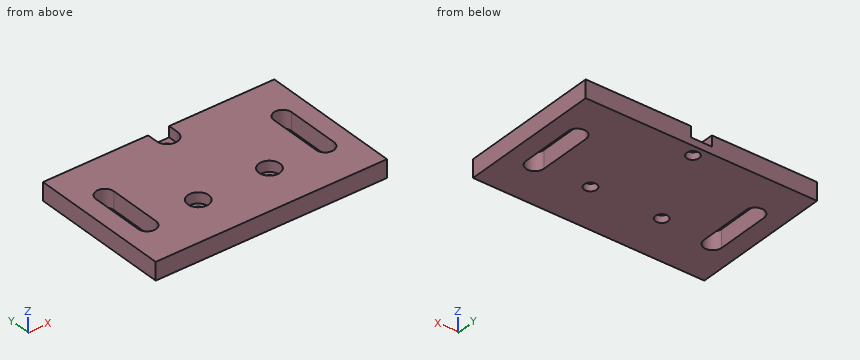
from build123d import *

# Parameters (mm, degrees)
F0_W     = 65
F0_H     = 40
F0_R     = 1.75
F1_DEPTH = 5
F2_R     = 2.95
F2_R_2   = 1.75
F3_DEPTH = 3


with BuildPart() as f1:
    # F0 (on Top) → F1 (new body)
    with BuildSketch(Plane.XY):
        Rectangle(F0_W, F0_H)
        with Locations((-10, -6.7)):
            Circle(F0_R, mode=Mode.SUBTRACT)
        with Locations((10, -6.7)):
            Circle(F0_R, mode=Mode.SUBTRACT)
        with BuildLine():
            ThreePointArc((-22.5, -7.5), (-25, -10), (-27.5, -7.5))
            Line((-27.5, -7.5), (-27.5, 7.5))
            ThreePointArc((-27.5, 7.5), (-25, 10), (-22.5, 7.5))
            Line((-22.5, 7.5), (-22.5, -7.5))
        make_face(mode=Mode.SUBTRACT)
        with BuildLine():
            ThreePointArc((27.5, -7.5), (25, -10), (22.5, -7.5))
            Line((22.5, -7.5), (22.5, 7.5))
            ThreePointArc((22.5, 7.5), (25, 10), (27.5, 7.5))
            Line((27.5, 7.5), (27.5, -7.5))
        make_face(mode=Mode.SUBTRACT)
        with Locations((0, 17)):
            Circle(F0_R, mode=Mode.SUBTRACT)
    extrude(amount=F1_DEPTH)

    # F2 (on face) → F3 (cut)
    with BuildSketch(Plane.XY.offset(5)):
        with Locations((10, -6.7)):
            Circle(F2_R)
        with Locations((10, -6.7)):
            Circle(F2_R_2, mode=Mode.SUBTRACT)
        with Locations((-10, -6.7)):
            Circle(F2_R_2)
        with Locations((-10, -6.7)):
            Circle(F2_R)
        with Locations((-10, -6.7)):
            Circle(F2_R_2, mode=Mode.SUBTRACT)
        with BuildLine():
            Line((-2.949923, 20), (-2.949923, 17.021281))
            ThreePointArc((-2.949923, 17.021281), (0, 14.05), (2.949923, 17.021281))
            Line((2.949923, 17.021281), (2.949923, 20))
            Line((2.949923, 20), (-2.949923, 20))
        make_face()
        with Locations((0, 17)):
            Circle(F2_R_2, mode=Mode.SUBTRACT)
    extrude(amount=-F3_DEPTH, mode=Mode.SUBTRACT)


solid = f1.part
Can you work these out from the model? Positions are in its coordinate system, mm. Coordinates: 2 decimals unless noted, no trailing zeros. Loops run counter-clockwise (first coordinate to the right, second up) from the corner with the lowest first, then second, coordinate; pieces in that order, holes last. Notation, with made-up numbers: (63, -23.75) - (97, -23.75) arc R19 cw to (97, -7.75) - close; hole circle Ø6 at (52.25, 54.5). An arc over 180 degrees is marked (long way). Answer as a JSON object with one key per item and string values. Group by question number.
Item 1: If we section it at D-D (z = 4.3): List the corners of the cut face in (x, y) for me, plus the area to 3 significant figures.
Item 2: For pin 1 (1.8 mm diameter, centred on x = -1, y = 15.5, fed in from +Z), with a flat end and sliding along its axis, tell me the tip position at first contact or that it passes through.
Item 3: If I drill on L1, parallel to X at y = 6.5, z = 2.5; L2, parallel to Y at x = -10, z = 3.4; L3, parallel to Y at x = 10, z = 0.9, over which ranges is the centre line in solid material (lowest first)? Write a range as from..to.
Item 4: If we section it at B-B (x = 0): List the corners of the cut face in (y, z) for me, plus the area to 3 significant figures.
Item 5: If we section it at C-C (y = 6): List the corners of the cut face in (x, z) for me, plus the area to 3 significant figures.
Item 6: If we section it at A-A (y = -6.7): List the corners of the cut face in (x, z) for me.
Returned:
{
 "1": {"outline": "(-32.5, -20) - (32.5, -20) - (32.5, 20) - (2.95, 20) - (2.95, 17.02) arc R2.95 cw (long way) to (-2.95, 17.02) - (-2.95, 20) - (-32.5, 20) - close; hole (-27.5, -7.5) arc R2.5 ccw to (-22.5, -7.5) - (-22.5, 7.5) arc R2.5 ccw to (-27.5, 7.5) - close; hole circle Ø5.9 at (-10, -6.7); hole circle Ø5.9 at (10, -6.7); hole (22.5, -7.5) arc R2.5 ccw to (27.5, -7.5) - (27.5, 7.5) arc R2.5 ccw to (22.5, 7.5) - close", "area": "2,320 mm²"},
 "2": {"pin 1": "stops at z = 2"},
 "3": {"L1": "x = -32.5..-27.5, -22.5..22.5, 27.5..32.5", "L2": "y = -20..-9.65, -3.75..20", "L3": "y = -20..-8.45, -4.95..20"},
 "4": {"outline": "(-20, 0) - (15.25, 0) - (15.25, 2) - (14.05, 2) - (14.05, 5) - (-20, 5) - close; (18.75, 0) - (20, 0) - (20, 2) - (18.75, 2) - close", "area": "175 mm²"},
 "5": {"outline": "(-32.5, 0) - (-27.5, 0) - (-27.5, 5) - (-32.5, 5) - close; (-22.5, 0) - (22.5, 0) - (22.5, 5) - (-22.5, 5) - close; (27.5, 0) - (32.5, 0) - (32.5, 5) - (27.5, 5) - close", "area": "275 mm²"},
 "6": {"outline": "(-32.5, 0) - (-27.5, 0) - (-27.5, 5) - (-32.5, 5) - close; (-22.5, 0) - (-11.75, 0) - (-11.75, 2) - (-12.95, 2) - (-12.95, 5) - (-22.5, 5) - close; (-8.25, 0) - (8.25, 0) - (8.25, 2) - (7.05, 2) - (7.05, 5) - (-7.05, 5) - (-7.05, 2) - (-8.25, 2) - close; (11.75, 0) - (22.5, 0) - (22.5, 5) - (12.95, 5) - (12.95, 2) - (11.75, 2) - close; (27.5, 0) - (32.5, 0) - (32.5, 5) - (27.5, 5) - close"}
}
